Can you work these out from the model? Positions are in its coordinate system, mm. Face numbers are marked on the shaded views. A direction names the side the tool comes from. Give positions to 0.01 mm unless a question says otherwise; leave off trailing zeros. Loops run counter-clockwise (first coordinate to the right, second up) from the corner with the lowest first, then second, coordinate; pieces in that order, holes last. Notation, with made-up numbers: (62, -36.75) -> (87, -36.75) arc R11 cw to (87, -24.75) -> close; hole circle Ø4 at (69, 86). An arc over 180 degrees is marked (long way). One line per question, with ' | ' between items.
Autodesk Inventor part; units mm, degrees
ref_plane "YZ Plane" through (0, 0, 0) normal (1, 0, 0) x (0, 1, 0)
ref_plane "XZ Plane" through (0, 0, 0) normal (0, 1, 0) x (-1, 0, 0)
ref_plane "XY Plane" through (0, 0, 0) normal (0, 0, 1) x (1, 0, 0)
sketch "Sketch1" plane through (0, 0, 0) normal (0, 1, 0) x (-1, 0, 0)
  line L0 (20.25, -10) -> (-20.25, -10)
  line L1 (-20.25, -10) -> (-20.25, 10)
  line L2 (-20.25, 10) -> (20.25, 10)
  line L3 (20.25, 10) -> (20.25, -10)
  point P0 (0, 0)
  dimension "d0" = 40.5
  dimension "d1" = 20
  dimension "d2" = 10
  dimension "d3" = 20.25
extrude "Plate1" add sketch "Sketch1" along normal blind 1.5
sketch "Sketch2" plane through (21.75, 0, -10) normal (-1, 0, 0) x (0, -1, 0)
  line L0 (0, 20) -> (0, 0)
  line L1 (0, 0) -> (-45, 0)
  line L2 (-45, 0) -> (-45, 20)
  line L3 (-45, 20) -> (0, 20)
edge flange "Flange1" height 45 angle 90 thickness 1.5 bend radius 0.31 thickness toward (-1, 0, 0) relief tear relief width 1.5 relief depth 0.75 edges at (20.25, 1.5, 0) wall of the first edge with corners at (21.75, 0, 10) (21.75, 0, -10) (21.75, 45, -10) (21.75, 45, 10)
bend "Bend1"
corner "Corner1"
sketch "Sketch3" plane through (-21.75, 0, 10) normal (1, 0, 0) x (0, 1, 0)
  line L0 (0, -20) -> (0, 0)
  line L1 (0, 0) -> (45, 0)
  line L2 (45, 0) -> (45, -20)
  line L3 (45, -20) -> (0, -20)
edge flange "Flange2" height 45 angle 90 thickness 1.5 bend radius 0.31 thickness toward (1, 0, 0) relief tear relief width 1.5 relief depth 0.75 edges at (-20.25, 1.5, 0) wall of the first edge with corners at (-21.75, 0, -10) (-21.75, 0, 10) (-21.75, 45, 10) (-21.75, 45, -10)
bend "Bend2"
corner "Corner2"
sketch "Sketch4" plane through (21.75, 45, 10) normal (1, 0, 0) x (0, 0, -1)
  circle A0 centre (10, -9.9) radius 6.75
  line L0 (0, 0) -> (20, 0)
  line L1 (20, 0) -> (20, -43.19)
  point P0 (10, -45)
  dimension "d25" = 9.9
  dimension "d26" = 13.5
  dimension "d27" = 10
extrude "Extrusion1" cut sketch "Sketch4" against normal blind 50
sketch "Sketch5" plane through (21.75, 45, 10) normal (1, 0, 0) x (0, 0, -1)
  circle A0 centre (10, -9.9) radius 6.75
  line L0 (0, 0) -> (20, 0)
  line L1 (-4, 0) -> (24, 0)
  line L2 (24, 0) -> (24, -9.9)
  line L3 (24, -9.9) -> (-4, -9.9)
  line L4 (-4, -9.9) -> (-4, 0)
  line L5 (0, -43.19) -> (0, 0)
  point P0 (10, -45)
  dimension "d30" = 9.9
  dimension "d31" = 28
  dimension "d32" = 4
extrude "Extrusion2" cut sketch "Sketch5" against normal blind 50 contours L3 A0 | A0 L3 L5 L0 L1 L2 | L3 L4 L1 L5 picked at (11.6841, -8.408)
fillet "Fillet1" radius 1 4 edges at (-21, 35.1, 10) (-21, 35.1, -10) (21, 35.1, -10) (21, 35.1, 10)
sketch "Sketch8" plane through (0, 0, 0) normal (0, -1, 0) x (1, 0, 0)
  circle A0 centre (8, -8) radius 1.05
  circle A1 centre (-8, -8) radius 1.05
  circle A2 centre (8, 8) radius 1.05
  circle A3 centre (-8, 8) radius 1.05
  circle A4 centre (-7, -7) radius 1.5
  line L0 (-9.33, -10.07) -> (7.53, -10.07)
  line L1 (10.07, -8.5) -> (10.07, 29.6)
  circle A5 centre (7, -7) radius 1.5
  circle A6 centre (-7, 7) radius 1.5
  circle A7 centre (7, 7) radius 1.5
  point P0 (0, 0)
  dimension "d71" = 7
  dimension "d72" = 7
  dimension "d73" = 3
  dimension "d76" = 14
  dimension "d79" = 14
hole "Hole3" at (-7, 0, -7) at (-7, 0, 7) at (7, 0, 7) at (7, 0, -7) direction (0, 1, 0) diameter 3 depth 1.5
sketch "Sketch9" plane through (-21.75, 1.81, -10) normal (-1, 0, 0) x (0, 0, 1)
  circle A0 centre (17.525, 20.79) radius 0.7835
  circle A1 centre (17.525, 5.69) radius 0.7835
  circle A2 centre (2.475, 20.79) radius 0.7835
  circle A3 centre (2.475, 5.69) radius 0.7835
  point P0 (10, -1.81)
hole "Hole4" at (-21.75, 7.5, 7.525) at (-21.75, 7.5, -7.525) at (-21.75, 22.6, -7.525) at (-21.75, 22.6, 7.525) direction (1, 0, 0) diameter 2.1 depth 1.5
sketch "Sketch10" plane through (21.75, 1.81, 10) normal (1, 0, 0) x (0, 0, -1)
  circle A0 centre (3, 13.17) radius 0.7835
  circle A1 centre (10, 5.87) radius 0.7835
  circle A2 centre (17, 13.17) radius 0.7835
  circle A3 centre (2, 26.39) radius 0.7835
  circle A4 centre (18, 26.39) radius 0.7835
  point P0 (10, -1.81)
hole "Hole5" at (21.75, 28.2, 8) at (21.75, 28.2, -8) at (21.75, 14.98, -7) at (21.75, 7.68, 0) at (21.75, 14.98, 7) direction (-1, 0, 0) diameter 2.1 depth 1.5
equation "\"d55\" = Thickness"
equation "\"d62\" = Thickness"
equation "\"d69\" = Thickness"
equation "\"d4\" = Thickness"
equation "\"d5\" = BendReliefWidth"
equation "\"d6\" = BendReliefDepth"
equation "\"d7\" = MinimumRemnant"
equation "\"d8\" = TransitionRadius"
equation "\"d11\" = BendRadius"
equation "\"d12\" = CornerReliefSize"
equation "\"d13\" = GapSize"
equation "\"d14\" = JacobiRadiusSize"
equation "\"d15\" = BendReliefWidth"
equation "\"d16\" = BendReliefDepth"
equation "\"d17\" = MinimumRemnant"
equation "\"d18\" = TransitionRadius"
equation "\"d21\" = BendRadius"
equation "\"d22\" = CornerReliefSize"
equation "\"d23\" = GapSize"
equation "\"d24\" = JacobiRadiusSize"
equation "\"BendReliefWidth\" = Thickness"
equation "\"BendReliefDepth\" = 0.5 * Thickness"
equation "\"CornerReliefSize\" = 4 * Thickness"
equation "\"MinimumRemnant\" = 2 * Thickness"
equation "\"TransitionRadius\" = BendRadius"
equation "\"JacobiRadiusSize\" = BendRadius"
equation "\"GapSize\" = Thickness"
properties part number "axis_10_top_frame" material "Aluminum 6061-AHC"
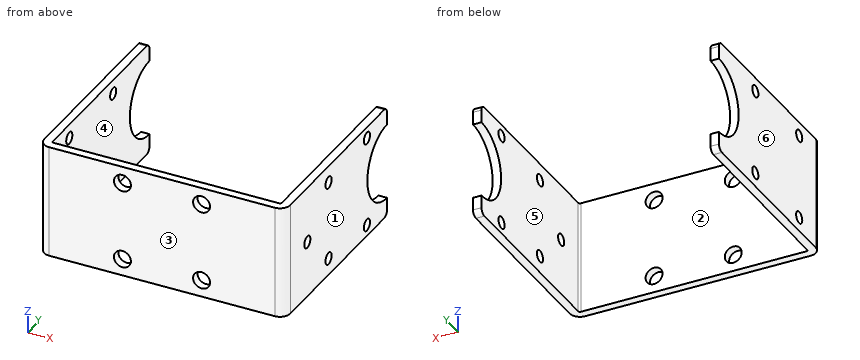
Q1. If we section it at D-D (z = 1.75): Write out the boundary of the cut face in (x, y).
Entries:
outline: (-21.75, 1.81) arc R1.81 ccw to (-19.94, 0) -> (19.94, 0) arc R1.81 ccw to (21.75, 1.81) -> (21.75, 28.58) -> (20.25, 28.58) -> (20.25, 1.81) arc R0.31 cw to (19.94, 1.5) -> (-19.94, 1.5) arc R0.31 cw to (-20.25, 1.81) -> (-20.25, 28.58) -> (-21.75, 28.58) -> close
Q2. For pin 1 Ø10 at (x, z) = (-5, 2.5) entering from +Y; pin 2 Ø1.9 at (y, z) = (7.5, 7.525) entering from -X; pin 3 Ø2.5 at (x, z) = (7, 7) entering from +Y, each with a flat end and sliding along its axis, tell me the tip position at first contact or that it passes through.
Entries:
pin 1: y = 1.5 | pin 2: x = 20.25 | pin 3: through
Q3. If we section it at B-B (y = 14.98): Write out the boundary of the cut face in (x, z), plus the area to 3 significant figures.
Entries:
outline: (-21.75, -10) -> (-20.25, -10) -> (-20.25, 10) -> (-21.75, 10) -> close; (20.25, -10) -> (21.75, -10) -> (21.75, -8.05) -> (20.25, -8.05) -> close; (20.25, -5.95) -> (21.75, -5.95) -> (21.75, 5.95) -> (20.25, 5.95) -> close; (20.25, 8.05) -> (21.75, 8.05) -> (21.75, 10) -> (20.25, 10) -> close | area: 53.7 mm²
Q4. If we section it at C-C (y = 4.5): Write out the boundary of the cut face in (x, z).
Entries:
outline: (-21.75, -10) -> (-20.25, -10) -> (-20.25, 10) -> (-21.75, 10) -> close; (20.25, -10) -> (21.75, -10) -> (21.75, 10) -> (20.25, 10) -> close
Q5. On a 3-axis mill with a long thin cutter (end or side, diameter ignored), from which of +Z, -Z, +X, -X, +Y, -Y can I reach the whole of each face in a straight line? I mean the marked faces 5 and 6. Say none if no direction works.
Entries:
face 5: +Z, -Z, +Y | face 6: +Z, -Z, -X, +Y, -Y
Q6. If we section it at A-A (x = -7): Write out the boundary of the cut face in (y, z).
Entries:
outline: (0, -10) -> (1.5, -10) -> (1.5, -8.5) -> (0, -8.5) -> close; (0, -5.5) -> (1.5, -5.5) -> (1.5, 5.5) -> (0, 5.5) -> close; (0, 8.5) -> (1.5, 8.5) -> (1.5, 10) -> (0, 10) -> close
Q7. If we mould it in two halves opening along X, with no side actions, what happens to the marked faces 1, 2, 3 and 4? For each: pulls with the +X half, pulls with the -X half, needs draft (parallel to the pull), parting line crosses it, or undercut.
Entries:
face 1: pulls with the +X half | face 2: undercut | face 3: needs draft | face 4: undercut
Q8. If I drill on probe 1 along Z at (x, y) = (7, 0.8); probe 2 along X at (y, z) = (17, -0.75); probe 3 along Z at (x, y) = (21.25, 28.2), over which ranges is the centre line in solid material (lowest first)? Write a range as from..to.
Entries:
probe 1: -10..-8.5, -5.5..5.5, 8.5..10 | probe 2: -21.75..-20.25, 20.25..21.75 | probe 3: -10..-9.05, -6.95..6.95, 9.05..10
